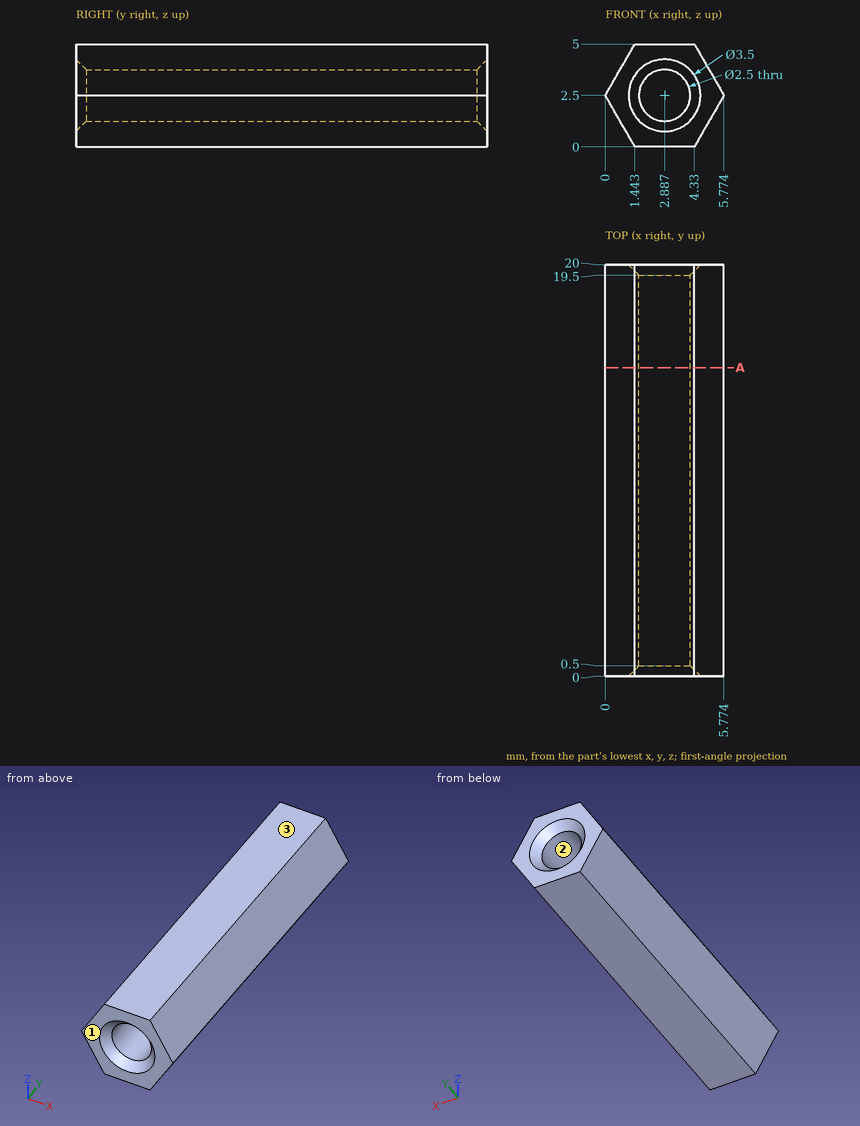
Verification items for this drawing (mm, ordinates from the low corner). Give positions to 0.01 mm unless a question says otherwise; leave off trailing zeros. Loops run counter-clockwise (first coordinate to the right, second up) from the corner with the lowest first, then second, coordinate; pieces in that order, holes last. Notation, with made-up numbers: M -36,75.5 L 22,75.5 A19 ccw 22,79.5 Z; hole C 71.5,12.25 d3. An arc over 180 degrees is marked long. Answer as a JSON object with one key per item and string values. Group by question number.
Q1. Release check for a two-part mould opening along Z. For the marked faces 1, 2 and 3 record: released by +Z, released by -Z, zero draft, split by the parting line, or undercut.
Q2. Cross-section at A-A on y = 15. Record the cut outline in (x, z).
Q3. Material ranges on line 1 along Z through (x, y) = (2.8, 1.25); line 2 along Z through (x, y) = (3.45, 6) (1 decimal); line 3 along Y through (x, z) = (1.8, 1.5) (1 decimal), recorded low to high. Write a range as [from, to].
Q4. Go/stop test with a flat-tipped pin: P1, Ø3, axis at x = 4.5, y = 10.5, coming from the -Z side. Record where the tip stops, or that it passes through.
Evaluation:
{
 "1": {"face 1": "zero draft", "face 2": "undercut", "face 3": "released by +Z"},
 "2": {"outline": "M 0,2.5 L 1.44,0 L 4.33,0 L 5.77,2.5 L 4.33,5 L 1.44,5 Z; hole C 2.89,2.5 d2.5"},
 "3": {"line 1": "z = [0, 1.25], [3.75, 5]", "line 2": "z = [0, 1.4], [3.6, 5]", "line 3": "y = [0.3, 19.7]"},
 "4": {"P1": "stops at z = 0"}
}
